Study the drawing (mm; zero at the part's minimum x, y, z) and answer. Round coordinates to 2 decimals unless told otherwise and drop trailing zeros. Write each loop counter-clockwise with the first axis right and the second up, starting at its lowest first coordinate (ties: lowest second). Pieces come first, ordered by that corner, then holes. Notation, with made-up numbers: M 18.25,-20 L 44.25,-20 A14 ccw 44.25,2 Z; hole C 28,-24.5 d3. An arc over 180 degrees is marked long. Write each question's results on one line, items separated by ' | '.
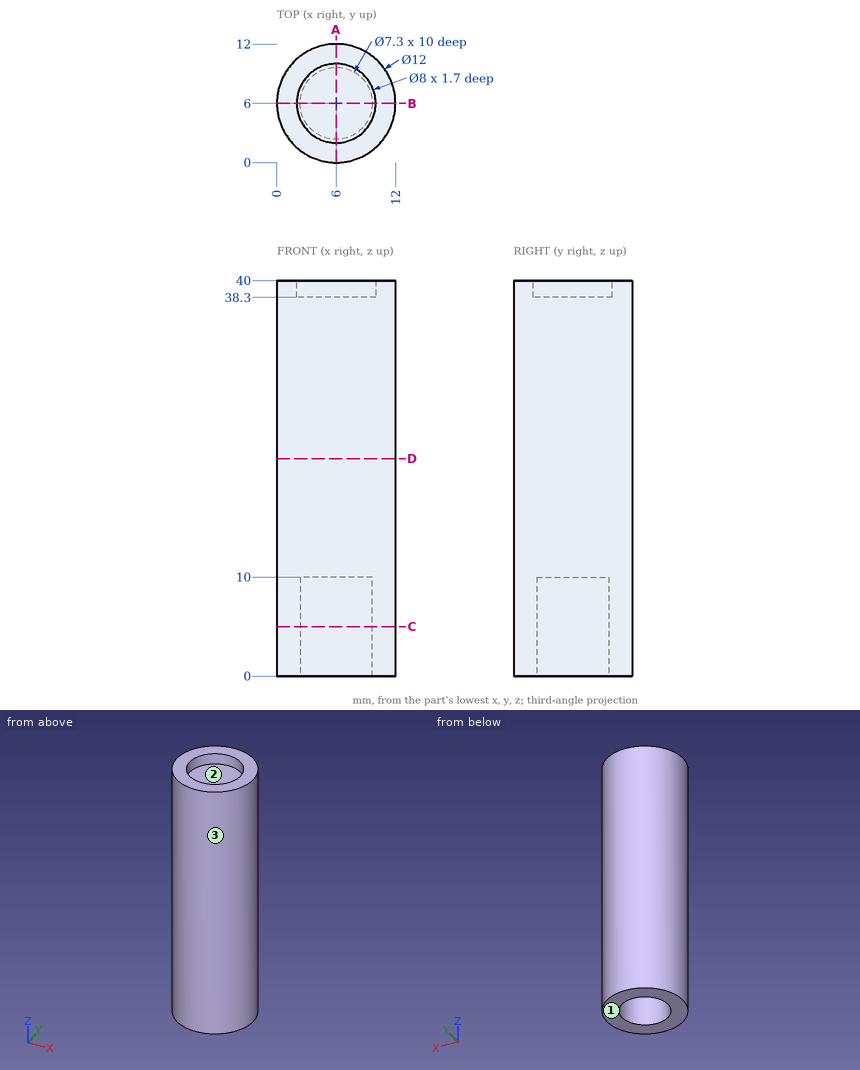
1) Each of these flat-tipped pins is pushed along its axis until it touches: pin 1 (7 mm diameter, centred on x = 6, y = 6, fed in from +Z); pin 2 (1.5 mm diameter, centred on x = 7.5, z = 28, fed in from +Y). Where does it stop, or does it pass through?
Return value:
pin 1: z = 38.3 | pin 2: y = 11.95
2) Find the intervals of material crossed by line 1 (Y direction, x = 6, z = 7); line 2 (Y direction, x = 6, z = 38.95); line 3 (Z direction, x = 4.75, y = 3), in increasing order.
Return value:
line 1: 0 to 2.35, 9.65 to 12 | line 2: 0 to 2, 10 to 12 | line 3: 10 to 38.3
3) Section D-D (z = 22) is taken. Determine the outline of the cut face in (x, y), then the cut area to 3 significant figures.
Return value:
outline: C 6,6 d12 | area: 113 mm²
4) Section C-C (z = 5) is taken. Determine the outline of the cut face in (x, y).
Return value:
outline: C 6,6 d12; hole C 6,6 d7.3
5) Section A-A (x = 6) is taken. Determine the outline of the cut face in (y, z), then the cut area to 3 significant figures.
Return value:
outline: M 0,0 L 2.35,0 L 2.35,10 L 9.65,10 L 9.65,0 L 12,0 L 12,40 L 10,40 L 10,38.3 L 2,38.3 L 2,40 L 0,40 Z | area: 393 mm²
6) The mould has two halves that part along Y. Classify the marked faces 1, 2 and 3: +Y half, -Y half, draft (parallel to the pull), parting line (faces both ways), or undercut.
Return value:
face 1: draft | face 2: undercut | face 3: parting line
